The figure shows three views and two pictorial views of one solid part (mm, origin at its lowest corner). Answer the questions. A direction names the side the tool comes from. Give positions to 0.01 mm unless a question says otherwise; leave off trailing zeros. Loops run counter-clockwise (first coordinate to the right, second up) from the corner with the lowest first, then second, coordinate; pieces in that order, holes last. Notation, with made-up numbers: M 86.5,12 L 134.5,12 A18 ccw 134.5,41 Z; hole C 49.25,4 d6. An arc over 180 degrees is marked long. Write item = value, one per line. Start each with the question number.
1. For the marked faces 1, 2, 3 and 4, determine the directions among +Z, -Z, +X, -X, +Y, -Y from which every point of the face is accessible in a straight line to the end or side of a thin tool.
2. Section A-A on x = 50 is taken. Determine the outline of the cut face in (y, z).
3. Section B-B on z = 28.5 is taken. Determine the outline of the cut face in (x, y), plus the area to 3 significant figures.
4. Flat-ended cylindrical pins translate along their axes: pin 1 Ø25 at (x, z) = (51, 39.5) entering from -Y; pin 2 Ø12 at (x, y) = (46, 21) entering from +Z; pin 3 Ø1 at (x, y) = (35.5, 45) entering from +Z; pin 4 Ø16 at (x, y) = (85, 49.5) entering from +Z. Find the tip coordinate at first contact, or state that the pin passes through.
5. Consider L1, parallel to Z at x = 12, y = 52; L2, parallel to Z at x = 34.5, y = 20.5; L3, parallel to Y at x = 37.5, z = 29. Determine where each line is inside the solid, lowest interval first. Write a range as [from, to].
6. Section D-D on x = 88 is taken. Determine the outline of the cut face in (y, z).
7. Section C-C on y = 44 is taken. Determine the outline of the cut face in (x, z).
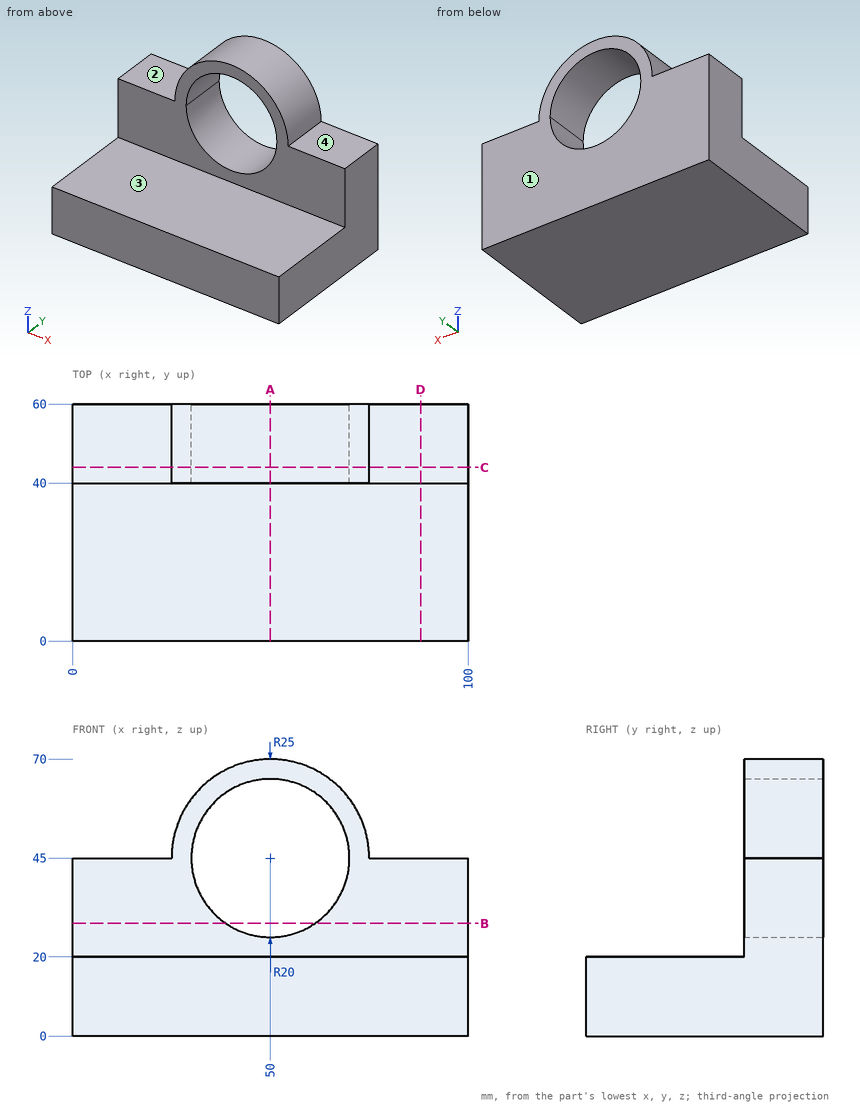
Verdict:
q1.face_1 = +Z, -Z, +X, -X, +Y
q1.face_2 = +Z, -X, +Y, -Y
q1.face_3 = +Z, +X, -X, -Y
q1.face_4 = +Z, +X, +Y, -Y
q2.outline = M 0,0 L 60,0 L 60,25 L 40,25 L 40,20 L 0,20 Z; M 40,65 L 60,65 L 60,70 L 40,70 Z
q3.outline = M 0,40 L 38.7,40 L 38.7,60 L 0,60 Z; M 61.3,40 L 100,40 L 100,60 L 61.3,60 Z
q3.area = 1,550 mm2
q4.pin_1 = through
q4.pin_2 = 20
q4.pin_3 = 65.71
q4.pin_4 = 45
q5.L1 = [0, 45]
q5.L2 = [0, 20]
q5.L3 = [40, 60]
q6.outline = M 0,0 L 60,0 L 60,45 L 40,45 L 40,20 L 0,20 Z
q7.outline = M 0,0 L 100,0 L 100,45 L 75,45 A25 ccw 25,45 L 0,45 Z; hole C 50,45 d40
